from build123d import *

# Parameters (mm, degrees)
F0_R     = 11
F1_DEPTH = 6
F2_SIZE  = 0.99999


# Not quite as in the source:
# - a fillet or chamfer is up to 0.001 mm smaller than in the source, because OpenCascade refuses the exact size


with BuildPart() as f1:
    # F0 (on Top) → F1 (new body)
    with BuildSketch(Plane.XY):
        with BuildLine():
            ThreePointArc((-8.3993012068, 20.8970612253), (4.6296691825, 37.9782845851), (0, 17))
            ThreePointArc((0, 17), (-10.3245446798, 13.5056942492), (-16.4047227892, 4.4592679005))
            ThreePointArc((-16.4047227892, 4.4592679005), (-18.5023983731, 1.580095835), (-21.984408769, 0.8281129622))
            ThreePointArc((-21.984408769, 0.8281129622), (-37.0912454672, -21.75043975), (-10.0741387442, -18.90728975))
            ThreePointArc((-10.0741387442, -18.90728975), (-10.1357694828, -18.1114057356), (-10.7602912032, -17.6142112737))
            Line((-10.7602912032, -17.6142112737), (-12.6979184167, -17.0950256266))
            ThreePointArc((-12.6979184167, -17.0950256266), (-13.420186678, -17.1748279717), (-13.8977352822, -17.7225388318))
            ThreePointArc((-13.8977352822, -17.7225388318), (-35.2049938341, -14.9797311694), (-14.7224318643, -8.5))
            ThreePointArc((-14.7224318643, -8.5), (-6.5340019757, -15.6941650999), (4.3405221105, -16.4365406278))
            ThreePointArc((4.3405221105, -16.4365406278), (7.882796053, -16.8135949396), (10.275037522, -19.4531129622))
            ThreePointArc((10.275037522, -19.4531129622), (37.3820561006, -21.2467409576), (21.4112626123, 0.7291848013))
            ThreePointArc((21.4112626123, 0.7291848013), (20.7528222067, 0.2778690088), (20.6345000323, -0.5115798972))
            Line((20.6345000323, -0.5115798972), (21.1536856793, -2.4492071107))
            ThreePointArc((21.1536856793, -2.4492071107), (21.5839306681, -3.0348086009), (22.297036489, -3.1745223935))
            ThreePointArc((22.297036489, -3.1745223935), (30.5753246516, -22.9985534157), (14.7224318643, -8.5))
            ThreePointArc((14.7224318643, -8.5), (16.8585466555, 2.1884708506), (12.0642006787, 11.9772727273))
            ThreePointArc((12.0642006787, 11.9772727273), (10.6196023201, 15.2334991046), (11.709371247, 18.625))
            ThreePointArc((11.709371247, 18.625), (-0.2908106334, 42.9971807076), (-11.3371238681, 18.1781049487))
            ThreePointArc((-11.3371238681, 18.1781049487), (-10.6170527239, 17.8335367268), (-9.8742088291, 18.1257911709))
            Line((-9.8742088291, 18.1257911709), (-8.4557672626, 19.5442327374))
            ThreePointArc((-8.4557672626, 19.5442327374), (-8.1637439901, 20.2096365726), (-8.3993012068, 20.8970612253))
        make_face()
        Circle(F0_R, mode=Mode.SUBTRACT)
    extrude(amount=F1_DEPTH)

    # F2 (size 1 in the source; OpenCascade refuses exactly that, so slightly less here)
    f2_edges = [f1.edges().sort_by_distance(p)[0] for p in [
        (-37.091245, -21.75044, 6),
        (37.382056, -21.246741, 0),
    ]]
    chamfer(f2_edges, length=F2_SIZE)


solid = f1.part
Part model, mm, in its own coordinate system. A direction names the side the tool comes from. Coordinates: 2 decimals unless noted, no trailing zeros. Order: outer loops, then holes, each group sorted by start corner. A loop starts at its lowest first (then second) coordinate and runs counter-clockwise, first axis right, second up. Notation, with made-up numbers: (-14, 55.5) - (18, 55.5) arc R21 ccw to (18, 89.5) - close; hole circle Ø11 at (13, 14.25). An arc over 180 degrees is marked (long way). Use CSV: the item, a comma, the result in double quotes.
Item 1: 3-axis set-ups, long thin cutter, end or side, ignore diameter. For faces 4 (the face through (16.88, 2.03, 2.97)), 5 (the face through (-9.533, 19.184, 5.507)), 6 (the face through (-10.2, 13.6, 3)): which of +Z, -Z, +X, -X, +Y, -Y reach the whole face in a straight line?
Solved:
face 4,"+Z, -Z"
face 5,"+Z"
face 6,"+Z, -Z, -X"
Item 2: Mould opens along X. For faces 1 (the face through (3, -11, 6)), 2 (the face through (20.9, -1.5, 3)), 3 (the face through (0, 43, 3)) say: +X half, -X half, draft (parallel to the pull), parting line (faces both ways), or undercut.
Solved:
face 1,"draft"
face 2,"undercut"
face 3,"parting line"
Item 3: Saw through at B-B on z = 3.5. Give the cut face in (x, y) (1 decimal).
Solved:
outline,"(-22, 0.8) arc R15 ccw (long way) to (-10.1, -18.9) arc R1 ccw to (-10.8, -17.6) - (-12.7, -17.1) arc R1 ccw to (-13.9, -17.7) arc R11 cw (long way) to (-14.7, -8.5) arc R17 ccw to (4.3, -16.4) arc R5 cw to (10.3, -19.5) arc R15 ccw (long way) to (21.4, 0.7) arc R1 ccw to (20.6, -0.5) - (21.2, -2.4) arc R1 ccw to (22.3, -3.2) arc R11 cw (long way) to (14.7, -8.5) arc R17 ccw to (12.1, 12) arc R5 cw to (11.7, 18.6) arc R15 ccw (long way) to (-11.3, 18.2) arc R1 ccw to (-9.9, 18.1) - (-8.5, 19.5) arc R1 ccw to (-8.4, 20.9) arc R11 cw (long way) to (0, 17) arc R17 ccw to (-16.4, 4.5) arc R5 cw to start; hole circle Ø22 at (0, 0)"
Item 4: Saw through at C-C on y = -14. Give the number of separate pieces and of enclosed holes in the cut face, and give its area (3 significant figures).
Solved:
separate pieces,"3"
enclosed holes,"0"
area,"179 mm²"
Item 5: Probe probe 1 along Y at (x, z) = (24.5, 3); probe 2 along Y at (x, z) = (-5, 4.5); probe 3 along X at (y, z) = (-14, 4). List the from-to ranges inside material, lowest first.
Solved:
probe 1,"y = -29 to -25, -3 to 1"
probe 2,"y = -16.25 to -9.8, 9.8 to 16.25, 37.8 to 42.14"
probe 3,"x = -39.25 to -35.25, -9.64 to 13.25, 35.25 to 39.25"
Item 6: Drop flat-ended pins along their axis: P1, Ø1.5, axis at y = 26.5, z = 1, coming from the +X side; P2, Ø2, axis at y = -3.5, z = 2.5, coming from the +X side; P3, Ø2, axis at x = 30.5, z = 4.5, coming from the -Y side. Give the stop position or say it passes through.
Solved:
P1,"stops at x = 14.98"
P2,"stops at x = 35.86"
P3,"stops at y = -28.05"
Item 7: Saw through at A-A on y = 28. Give the cut face in (x, z).
Solved:
outline,"(-15, 1) - (-14, 0) - (-12, 0) - (-11, 1) - (-11, 5) - (-12, 6) - (-14, 6) - (-15, 5) - close; (11, 1) - (12, 0) - (14, 0) - (15, 1) - (15, 5) - (14, 6) - (12, 6) - (11, 5) - close"
